CAD build for the part. Positions are in the model's coordinates, mm. A direction names the side the tool comes from. Give positions to 0.01 mm unless a question says otherwise; leave off trailing zeros. Loops run counter-clockwise (first coordinate to the right, second up) from the corner with the lowest first, then second, coordinate; pieces in that order, holes last. Notation, with made-up numbers: (70.25, -24.75) - (95.25, -24.75) arc R17 ccw to (95.25, -17.75) - close; hole circle Ø2 at (-10, -20). An arc over 180 degrees is marked (long way). Return JSON: item names as keys, results as strings.
from build123d import *

# Parameters (mm, degrees)
F0_W     = 25
F0_H     = 100
F1_DEPTH = 3
F2_R     = 1.5
F3_DEPTH = 3


with BuildPart() as f1:
    # F0 (on Top) → F1 (new body)
    with BuildSketch(Plane.XY):
        Rectangle(F0_W, F0_H)
    extrude(amount=F1_DEPTH)

    # F2 (on face) → F3 (join)
    with BuildSketch(Plane.YZ.offset(12.5)):
        with BuildLine():
            Line((35, 9), (35, 3))
            Line((35, 3), (45, 3))
            Line((45, 3), (45, 9))
            ThreePointArc((45, 9), (43.828427, 11.828427), (41, 13))
            Line((41, 13), (39, 13))
            ThreePointArc((39, 13), (36.171573, 11.828427), (35, 9))
        make_face()
        with Locations((40, 8)):
            Circle(F2_R, mode=Mode.SUBTRACT)
        with BuildLine():
            Line((-45, 9), (-45, 3))
            Line((-45, 3), (-35, 3))
            Line((-35, 3), (-35, 9))
            ThreePointArc((-35, 9), (-36.171573, 11.828427), (-39, 13))
            Line((-39, 13), (-41, 13))
            ThreePointArc((-41, 13), (-43.828427, 11.828427), (-45, 9))
        make_face()
        with Locations((-40, 8)):
            Circle(F2_R, mode=Mode.SUBTRACT)
    extrude(amount=-F3_DEPTH)

    # F4: F1 across face


with BuildPart() as f1_1:
    add(f1.part)
    add(f1.part.mirror(Plane(origin=(-12.5, 0, 1.5), x_dir=(0, -1, 0), z_dir=(-1, 0, 0))))


solid = f1_1.part
1. Cut at D-D, the plane x = -26. Write the cut outline in (y, z).
Values follow:
{"outline": "(-50, 0) - (50, 0) - (50, 3) - (-50, 3) - close"}
2. Drop flat-ended pins along their axis: P1, Ø4, axis at x = -5.5, z = 4.5, coming from the +Y side; P2, Ø3.5, axis at x = 10.5, z = 6.5, coming from the +Y side; P3, Ø0.9, axis at x = 10.5, z = 6.5, coming from the -Y side; P4, Ø1.5, axis at x = -10.5, y = 31.5, coming from the +Z side. Give the stop position or say it passes through.
Values follow:
{"P1": "stops at y = 50", "P2": "stops at y = 45", "P3": "stops at y = -45", "P4": "stops at z = 3"}
3. Cut at B-B, the plane y = -40. Write the cut outline in (x, z).
Values follow:
{"outline": "(-37.5, 0) - (12.5, 0) - (12.5, 6.5) - (9.5, 6.5) - (9.5, 3) - (-34.5, 3) - (-34.5, 6.5) - (-37.5, 6.5) - close; (-37.5, 9.5) - (-34.5, 9.5) - (-34.5, 13) - (-37.5, 13) - close; (9.5, 9.5) - (12.5, 9.5) - (12.5, 13) - (9.5, 13) - close"}
4. Pull direction X, two halves, no side cores. Call faces 4 (the face through (-34.5, 38.8, 9.2)), 5 (the face through (12.5, 0, 2)), 6 (the face through (-36.021, 43.859, 11.797)): +X half, -X half, draft (parallel to the pull), parting line (faces both ways), or undercut.
Values follow:
{"face 4": "undercut", "face 5": "+X half", "face 6": "draft"}
5. Cut at C-C, the plane y = -10. Write the cut outline in (x, z), plus the area to 3 significant figures.
Values follow:
{"outline": "(-37.5, 0) - (12.5, 0) - (12.5, 3) - (-37.5, 3) - close", "area": "150 mm²"}
6. Drill centre lines: probe 1 along Y at (x, z) = (-35, 8.25); probe 2 along Z at (x, y) = (-35.8, 40); probe 3 along X at (y, z) = (36, 11.5). Where is each one in solid material? Low to high.
Values follow:
{"probe 1": "y = -45 to -41.48, -38.52 to -35, 35 to 38.52, 41.48 to 45", "probe 2": "z = 0 to 6.5, 9.5 to 13", "probe 3": "x = -37.5 to -34.5, 9.5 to 12.5"}
7. Which spindle directions (+Z, -Z, +X, -X, +Y, -Y) get a long thin tool onto all of the face, cutting with end or side? Do faces 1 (the face through (-36, -45, 6)), 2 (the face through (11, -35, 6)), 3 (the face through (9.5, 38.8, 9.2)). Say none if no direction does.
Values follow:
{"face 1": "+Z, +X, -X, -Y", "face 2": "+Z, +X, -X", "face 3": "+Z, +Y, -Y"}
8. Cut at A-A, the plane z = 8. Give the number of separate pieces and of enclosed holes in the cut face, plus the area to 3 significant figures.
Values follow:
{"separate pieces": "8", "enclosed holes": "0", "area": "84.0 mm²"}
